Autodesk Inventor part; units mm, degrees
ref_plane "YZ Plane" through (0, 0, 0) normal (1, 0, 0) x (0, 1, 0)
ref_plane "XZ Plane" through (0, 0, 0) normal (0, 1, 0) x (-1, 0, 0)
ref_plane "XY Plane" through (0, 0, 0) normal (0, 0, 1) x (1, 0, 0)
sketch "Sketch1" plane through (0, 0, 0) normal (0, 1, 0) x (-1, 0, 0)
  line L0 (5.5, -5.5) -> (-5.5, -5.5)
  line L1 (-5.5, -5.5) -> (-5.5, 5.5)
  line L2 (-5.5, 5.5) -> (5.5, 5.5)
  line L3 (5.5, 5.5) -> (5.5, -5.5)
  line L4 (5.5, -5.5) -> (-5.5, 5.5) construction
  line L5 (-5.5, -5.5) -> (5.5, 5.5) construction
  point P0 (0, 0)
  dimension "d0" = 11
  dimension "d1" = 11
extrude "Extrusion1" add sketch "Sketch1" along normal blind 3.25
sketch "Sketch2" plane through (0, 0, 0) normal (0, -1, 0) x (1, 0, 0)
  line L0 (-4.5, 4.5) -> (4.5, 4.5)
  line L1 (4.5, 4.5) -> (4.5, -4.5)
  line L2 (4.5, -4.5) -> (-4.5, -4.5)
  line L3 (-4.5, -4.5) -> (-4.5, 4.5)
  line L4 (-4.5, 4.5) -> (4.5, -4.5) construction
  line L5 (4.5, 4.5) -> (-4.5, -4.5) construction
  point P0 (0, 0)
  dimension "d4" = 9
  dimension "d5" = 9
extrude "Extrusion2" cut sketch "Sketch2" against normal blind 1
sketch "Sketch3" plane through (0, 3.25, 0) normal (0, 1, 0) x (1, 0, 0)
  line L0 (-4.75, -1.75) -> (-1.5, -1.75)
  line L1 (-1.5, -1.75) -> (-1.5, -4.75)
  line L2 (-1.5, -4.75) -> (-4.75, -4.75)
  line L3 (-4.75, -4.75) -> (-4.75, -1.75)
  line L4 (-4.75, -1.75) -> (-1.5, -4.75) construction
  line L5 (-1.5, -1.75) -> (-4.75, -4.75) construction
  line L6 (-5.5, 5.5) -> (-5.5, -5.5)
  line L7 (-5.5, -5.5) -> (5.5, -5.5)
  line L8 (-4.75, 4.75) -> (-1.5, 4.75)
  line L9 (-4.75, 1.75) -> (-4.75, 4.75)
  line L10 (-1.5, 4.75) -> (-4.75, 1.75) construction
  line L11 (-1.5, 1.75) -> (-4.75, 1.75)
  line L12 (-1.5, 4.75) -> (-1.5, 1.75)
  line L13 (1.5, -1.75) -> (4.75, -1.75)
  line L14 (1.5, -4.75) -> (1.5, -1.75)
  line L15 (4.75, -1.75) -> (1.5, -4.75) construction
  line L16 (4.75, -4.75) -> (1.5, -4.75)
  line L17 (4.75, -1.75) -> (4.75, -4.75)
  line L18 (1.5, 4.75) -> (4.75, 4.75)
  line L19 (1.5, 1.75) -> (1.5, 4.75)
  line L20 (4.75, 4.75) -> (1.5, 1.75) construction
  line L21 (4.75, 1.75) -> (1.5, 1.75)
  line L22 (4.75, 4.75) -> (4.75, 1.75)
  point P0 (0, 0)
  point P1 (-3.125, -3.25)
  point P2 (-3.125, 3.25)
  point P3 (3.125, -3.25)
  point P4 (3.125, 3.25)
  dimension "d8" = 3.25
  dimension "d9" = 3
  dimension "d10" = 0.75
  dimension "d11" = 0.75
  dimension "d14" = 6.5
  dimension "d17" = 6.25
extrude "Extrusion3" add sketch "Sketch3" along normal blind 6.5
properties material "Brass, Soft Yellow, Welded"
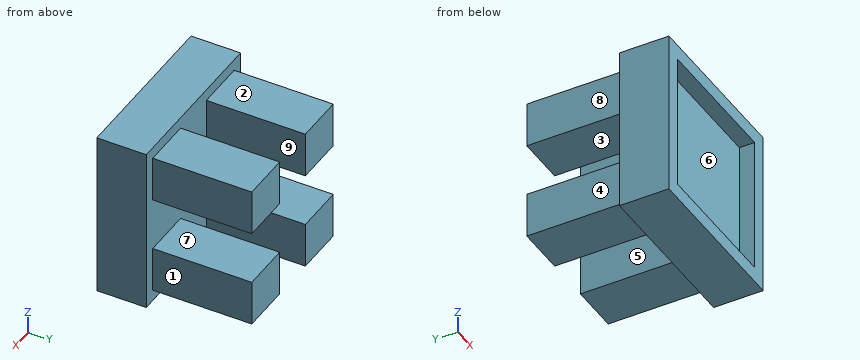
Can you work these out from the model? Positions are in its coordinate system, mm. Face numbers are marked on the shaded views. A direction names the side the tool comes from. Give positions to 0.01 mm unless a question says otherwise; leave off trailing zeros. Loops run counter-clockwise (first coordinate to the right, second up) from the corner with the lowest first, then second, coordinate; pieces in that order, holes last. Notation, with made-up numbers: (-25, 7) -> (14, 7) arc R24 ccw to (14, 26) -> close; hole circle Ø1 at (-16, -29). An arc over 180 degrees is marked (long way). Return JSON: item names as keys, results as strings.
Q1. For pin 1 Ø4 at (x, y) = (-1, 5) entering from +Z; pin 2 Ø3.5 at (y, z) = (7, 4) entering from -X; pin 3 Ø2.5 at (y, z) = (6, -2.5) entering from +X; pin 4 Ø2.5 at (x, y) = (-3, 7) entering from +Z, each with a flat end and sliding along its axis, tell me the tip position at first contact or that it passes through.
Checks:
{"pin 1": "stops at z = 5.5", "pin 2": "stops at x = -4.75", "pin 3": "stops at x = 4.75", "pin 4": "stops at z = 4.75"}
Q2. I want a section at D-D, the plane x = -0.5. List the corners of the cut face in (y, z) for me, then the cut area to 4 significant figures.
Checks:
{"outline": "(0, -5.5) -> (3.25, -5.5) -> (3.25, 5.5) -> (0, 5.5) -> (0, 4.5) -> (1, 4.5) -> (1, -4.5) -> (0, -4.5) -> close", "area": "26.75 mm2"}
Q3. We'd pull the mould along X, two halves only. Please class the marked faces 6, 7, 8 and 9: released by +X, released by -X, zero draft, split by the parting line, or undercut.
Checks:
{"face 6": "undercut", "face 7": "zero draft", "face 8": "released by -X", "face 9": "undercut"}
Q4. On a 3-axis mill with a long thin cutter (end or side, diameter ignored), from which of +Z, -Z, +X, -X, +Y, -Y can I reach the whole of each face in a straight line? I mean the marked faces 1, 2, 3, 4 and 5. Say none if no direction works.
Checks:
{"face 1": "+Z, -Z, +X, +Y", "face 2": "+Z, +X, -X, +Y", "face 3": "+X, -X, +Y", "face 4": "+Z, -Z, -X, +Y", "face 5": "+Z, -Z, +Y"}
Q5. I need wall thicknesses on probe 1 along X at (y, z) = (8.5, 2.5); probe 2 along Z at (x, y) = (2.5, 8.25); probe 3 along Y at (x, z) = (1, 4). Which ranges of each line are inside material? Lowest first, please.
Checks:
{"probe 1": "x = -4.75 to -1.5, 1.5 to 4.75", "probe 2": "z = -4.75 to -1.75, 1.75 to 4.75", "probe 3": "y = 1 to 3.25"}
Q6. I want a section at C-C, the plane x = -1.75. List the corners of the cut face in (y, z) for me.
Checks:
{"outline": "(0, -5.5) -> (3.25, -5.5) -> (3.25, -4.75) -> (9.75, -4.75) -> (9.75, -1.75) -> (3.25, -1.75) -> (3.25, 1.75) -> (9.75, 1.75) -> (9.75, 4.75) -> (3.25, 4.75) -> (3.25, 5.5) -> (0, 5.5) -> (0, 4.5) -> (1, 4.5) -> (1, -4.5) -> (0, -4.5) -> close"}
Q7. I want a section at B-B, the plane z = 2.5. List the corners of the cut face in (x, y) for me, then the cut area to 3 significant figures.
Checks:
{"outline": "(-5.5, 0) -> (-4.5, 0) -> (-4.5, 1) -> (4.5, 1) -> (4.5, 0) -> (5.5, 0) -> (5.5, 3.25) -> (4.75, 3.25) -> (4.75, 9.75) -> (1.5, 9.75) -> (1.5, 3.25) -> (-1.5, 3.25) -> (-1.5, 9.75) -> (-4.75, 9.75) -> (-4.75, 3.25) -> (-5.5, 3.25) -> close", "area": "69.0 mm2"}
Q8. I want a section at A-A, the plane y = 5. List the corners of the cut face in (x, z) for me.
Checks:
{"outline": "(-4.75, -4.75) -> (-1.5, -4.75) -> (-1.5, -1.75) -> (-4.75, -1.75) -> close; (-4.75, 1.75) -> (-1.5, 1.75) -> (-1.5, 4.75) -> (-4.75, 4.75) -> close; (1.5, -4.75) -> (4.75, -4.75) -> (4.75, -1.75) -> (1.5, -1.75) -> close; (1.5, 1.75) -> (4.75, 1.75) -> (4.75, 4.75) -> (1.5, 4.75) -> close"}
